Build history of the part. All positions in model axes, mm. A direction names the side the tool comes from. Coordinates: 2 decimals unless noted, no trailing zeros. Order: outer loops, then holes, each group sorted by start corner. A loop starts at its lowest first (then second) coordinate and runs counter-clockwise, first axis right, second up. Notation, with made-up numbers: (10.25, 22) - (53.25, 22) arc R34 ccw to (53.25, 60) - close; hole circle Ø11 at (64, 6.25). An arc over 180 degrees is marked (long way). One line per item, written item: value.
from build123d import *

# Parameters (mm, degrees)
TORUS_R           = 1
CYLINDER001_R     = 17
CYLINDER001_DEPTH = 50
CHAMFER_SIZE      = 1
CYLINDER_R        = 2.4
CYLINDER_DEPTH    = 3.1
ARRAY_X_COUNT     = 2
ARRAY_X_PITCH     = 29.7
ARRAY_Y_COUNT     = 2
ARRAY_Y_PITCH     = 29.5
BOX_W             = 40
BOX_H             = 40
BOX_DEPTH         = 4
FILLET_R          = 3
FILLET001_R       = 3
FILLET002_R       = 3
FILLET003_R       = 3


with BuildPart() as torus:
    # Torus → Torus (revolve)
    with BuildSketch(Plane(origin=(20, 20, 50), x_dir=(1, 0, 0), z_dir=(0, -1, 0))):
        with Locations((12, 0)):
            Circle(TORUS_R)
    revolve(axis=Axis((20, 20, 50), (0, 0, 1)))


with BuildPart() as chamfer_body:
    # Cylinder001 → Cylinder001 (new body)
    with BuildSketch(Plane(origin=(20, 20, 0), x_dir=(1, 0, 0), z_dir=(0, 0, 1))):
        Circle(CYLINDER001_R)
    extrude(amount=CYLINDER001_DEPTH)

    # Chamfer
    chamfer_edges = [chamfer_body.edges().sort_by_distance(p)[0] for p in [
        (3, 20, 50),
    ]]
    chamfer(chamfer_edges, length=CHAMFER_SIZE)


with BuildPart() as array:
    # Cylinder → Cylinder (new body)
    with BuildSketch(Plane(origin=(5, 5, 1.1), x_dir=(1, 0, 0), z_dir=(0, 0, 1))):
        Circle(CYLINDER_R)
    extrude(amount=CYLINDER_DEPTH)

    # Array X: Array ×2


with BuildPart() as array_1:
    add(array.part)
    with Locations(*[(i * ARRAY_X_PITCH, 0, 0) for i in range(1, ARRAY_X_COUNT)]):
        add(array.part)

    # Array Y: Array ×2


with BuildPart() as array_2:
    add(array_1.part)
    with Locations(*[(0, i * ARRAY_Y_PITCH, 0) for i in range(1, ARRAY_Y_COUNT)]):
        add(array_1.part)


with BuildPart() as cut001:
    # Box → Box (new body)
    with BuildSketch(Plane.XY):
        with Locations((20, 20)):
            Rectangle(BOX_W, BOX_H)
    extrude(amount=BOX_DEPTH)

    # Fillet
    fillet_edges = [cut001.edges().sort_by_distance(p)[0] for p in [
        (0, 0, 2),
    ]]
    fillet(fillet_edges, radius=FILLET_R)

    # Fillet001
    fillet001_edges = [cut001.edges().sort_by_distance(p)[0] for p in [
        (40, 0, 2),
    ]]
    fillet(fillet001_edges, radius=FILLET001_R)

    # Fillet002
    fillet002_edges = [cut001.edges().sort_by_distance(p)[0] for p in [
        (40, 40, 2),
    ]]
    fillet(fillet002_edges, radius=FILLET002_R)

    # Fillet003
    fillet003_edges = [cut001.edges().sort_by_distance(p)[0] for p in [
        (0, 40, 2),
    ]]
    fillet(fillet003_edges, radius=FILLET003_R)

    # Cut: cut Array
    add(array_2.part, mode=Mode.SUBTRACT)

    # Fusion: union Chamfer body
    add(chamfer_body.part)

    # Cut001: cut Torus
    add(torus.part, mode=Mode.SUBTRACT)


solid = cut001.part
1. Flat gauge pins, fed straight in: P1, Ø2, axis at y = 18, z = 40.5, coming from the +X side; P2, Ø6, axis at y = 32.5, z = 24, coming from the -X side; P3, Ø8, axis at x = 22, z = 42.5, coming from the +Y side; P4, Ø6, axis at x = 34.7, y = 34.5, coming from the -Z side. Where does each tip first touch, or does it go through?
Values found:
P1: stops at x = 36.97
P2: stops at x = 5.9
P3: stops at y = 37
P4: stops at z = 0
2. Probe line 1 along X through (y, z) = (5, 2.3); line 2 along Y through (x, z) = (5, 3); line 3 along X through (y, z) = (34, 2). List the from-to ranges inside material, lowest first.
Values found:
line 1: x = 0 to 2.6, 7.4 to 32.3, 37.1 to 40
line 2: y = 0 to 2.6, 7.4 to 32.1, 36.9 to 40
line 3: x = 0 to 2.65, 7.35 to 32.35, 37.05 to 40
3. 3-axis set-ups, long thin cutter, end or side, ignore diameter. For faces 5 (the face through (0.86, 0.9, 2.03)), 6 (the face through (35, 5, 1.1)): which of +Z, -Z, +X, -X, +Y, -Y reach the whole face in a straight line?
Values found:
face 5: +Z, -Z, -X, -Y
face 6: +Z
4. Two-plate mould, pull along X, no slides. Class faces 1 (the face through (6.509, 9.656, 26.185)), 2 (the face through (39.14, 39.1, 2.03)), 3 (the face through (6.11, 32.37, 2.53)), 4 (the face through (0, 20, 2)): pulls with the +X half, pulls with the -X half, needs draft (parallel to the pull), parting line crosses it, or undercut.
Values found:
face 1: parting line crosses it
face 2: pulls with the +X half
face 3: undercut
face 4: pulls with the -X half
5. Band-saw the part on A-A, the plane z = 30. Give the cut face in (x, y), and give its area (3 significant figures).
Values found:
outline: circle Ø34 at (20, 20)
area: 908 mm2
